CAD build for the part. Positions are in the model's coordinates, mm. A direction names the side the tool comes from. Coordinates: 2 decimals unless noted, no trailing zeros. Loops run counter-clockwise (first coordinate to the right, second up) from the corner with the lowest first, then second, coordinate; pieces in that order, holes last. Notation, with made-up numbers: (46, 21.25) -> (94, 21.25) arc R13 ccw to (94, 42.25) -> close; hole circle Ø9 at (57, 40.25). An arc over 180 degrees is marked (long way). Write item = value, one per line. Start each with the question number.
(1) Pull direction Y, two halves, no side cores. Call faces 4 (the face through (0, 0, 0)), 5 (the face through (-29.17, 2.24, 2.17)), 6 (the face through (-4.336, 85.07, 19.524)): +Y half, -Y half, draft (parallel to the pull), parting line (faces both ways), or undercut.
(2) Band-saw the part on D-D (y = 43). Write the cut outline in (x, z).
(3) Band-saw the part on C-C (z = 0). Write the cut outline in (x, y), and give its area (3 significant figures).
(4) Band-saw the part on B-B (y = 12). Write the cut outline in (x, z).
(5) Drill centre lines: line 1 (Y direction, x = -17, z = 9); line 2 (X direction, y = 69, z = 0); line 3 (Y direction, x = -24, z = -7). Where is each one in solid material? Low to high. Write a range as from..to.
(6) Tool access for faces 1 (the face through (23.5, 18, 9)), 2 (the face through (-3.905, 50.745, -29.745)), 3 (the face through (-23.5, 18, -9)): list every direction of +Z, -Z, +X, -X, +Y, -Y with a clear straight run to the whole face (end or side of a thin tool).
(7) Band-saw the part on A-A (x = 0). Write the cut outline in (y, z).
(8) Flat gauge pins, fed straight in: P1, Ø4, axis at x = -16, y = 50, coming from the -Z side; P2, Ø3, axis at x = -27, z = -3.5, coming from the -Y side; P3, Ø5, axis at y = 58.5, z = 11.5, coming from the +X side. Where does each tip first touch, or does it go through?
```python
from build123d import *

# Parameters (mm, degrees)
SKETCH1_R           = 30
BOSS_EXTRUDE1_DEPTH = 90
SKETCH8_W           = 6.5
SKETCH8_H           = 29
CUT_EXTRUDE5_DEPTH  = 20
SKETCH5_R           = 10
BOSS_EXTRUDE3_DEPTH = 35
SKETCH7_R           = 20
CUT_EXTRUDE4_DEPTH  = 10
CHAMFER1_SIZE       = 6


with BuildPart() as part:
    # Sketch1 → Boss-Extrude1 (new body)
    with BuildSketch(Plane(origin=(0, 0, 0), x_dir=(1, 0, 0), z_dir=(0, 1, 0))):
        Circle(SKETCH1_R)
    extrude(amount=BOSS_EXTRUDE1_DEPTH)

    # Sketch8 → Cut-Extrude5 (cut, symmetric)
    with BuildSketch(Plane.XY):
        with Locations((-26.75, 14.5)):
            Rectangle(SKETCH8_W, SKETCH8_H)
        with Locations((26.75, 14.5)):
            Rectangle(SKETCH8_W, SKETCH8_H)
    extrude(amount=CUT_EXTRUDE5_DEPTH, both=True, mode=Mode.SUBTRACT)

    # Sketch5 → Boss-Extrude3 (add, symmetric)
    with BuildSketch(Plane(origin=(0, 0, 0), x_dir=(0, 0, -1), z_dir=(1, 0, 0))):
        with Locations((0, 12)):
            Circle(SKETCH5_R)
    extrude(amount=BOSS_EXTRUDE3_DEPTH, both=True)

    # Sketch7 → Cut-Extrude4 (cut)
    with BuildSketch(Plane(origin=(0, 90, 0), x_dir=(1, 0, 0), z_dir=(0, 1, 0))):
        Circle(SKETCH7_R)
    extrude(amount=-CUT_EXTRUDE4_DEPTH, mode=Mode.SUBTRACT)

    # Chamfer1
    chamfer1_edges = [part.edges().sort_by_distance(p)[0] for p in [
        (-30, 90, 0),
    ]]
    chamfer(chamfer1_edges, length=CHAMFER1_SIZE)


solid = part.part
```
Findings below:
q1.face_4 = -Y half
q1.face_5 = undercut
q1.face_6 = draft
q2.outline = circle Ø60 at (0, 0)
q3.outline = (-35, 2) -> (-23.5, 2) -> (-23.5, 0) -> (23.5, 0) -> (23.5, 2) -> (35, 2) -> (35, 22) -> (23.5, 22) -> (23.5, 29) -> (30, 29) -> (30, 84) -> (24, 90) -> (20, 90) -> (20, 80) -> (-20, 80) -> (-20, 90) -> (-24, 90) -> (-30, 84) -> (-30, 29) -> (-23.5, 29) -> (-23.5, 22) -> (-35, 22) -> close
q3.area = 5,050 mm²
q4.outline = (-35, -10) -> (-23.5, -10) -> (-23.5, -18.65) arc R30 ccw to (23.5, -18.65) -> (23.5, -10) -> (35, -10) -> (35, 10) -> (23.5, 10) -> (23.5, 18.65) arc R30 ccw to (-23.5, 18.65) -> (-23.5, 10) -> (-35, 10) -> close
q5.line_1 = 0..80
q5.line_2 = -30..30
q5.line_3 = 4.86..19.14, 29..89
q6.face_1 = +X
q6.face_2 = +Y
q6.face_3 = -X
q7.outline = (0, -30) -> (84, -30) -> (90, -24) -> (90, -20) -> (80, -20) -> (80, 20) -> (90, 20) -> (90, 24) -> (84, 30) -> (0, 30) -> close
q8.P1 = -26.53
q8.P2 = 2.2
q8.P3 = 28.62
